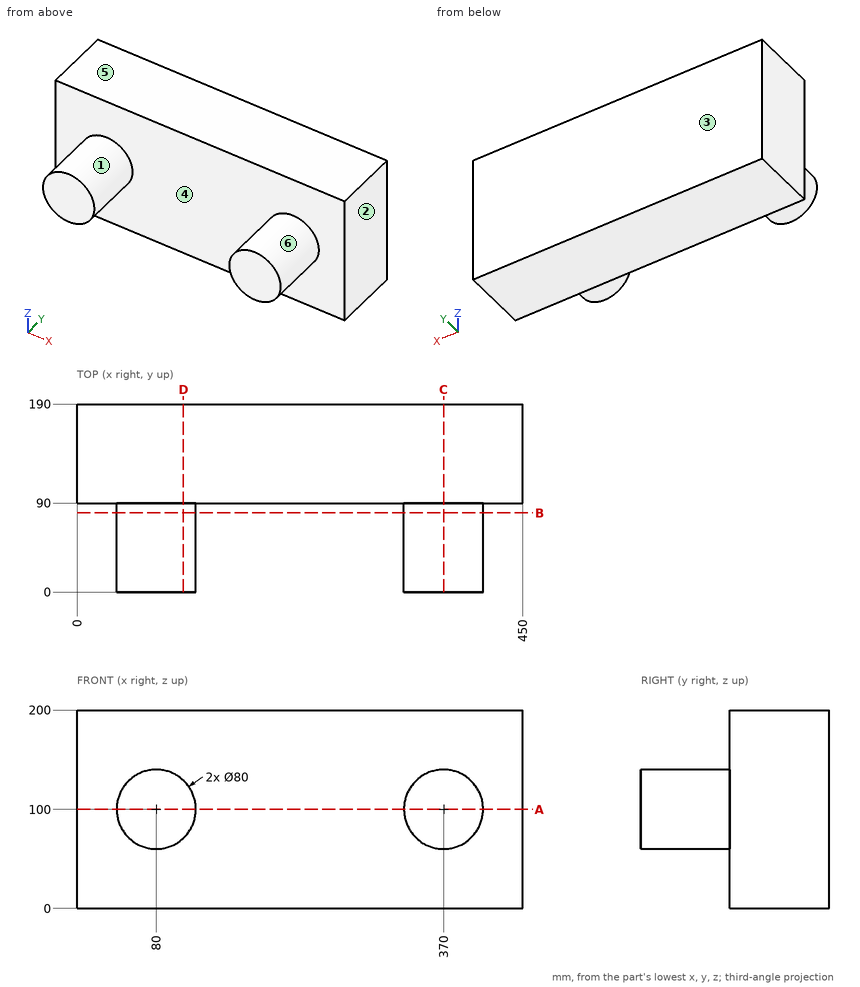
Answer from the drawing. Dimensions are ordinates in mm from the lowest x, y and z of the part. A direction names the side the tool comes from. Round coordinates to 2 decimals unless told otherwise and drop trailing zeros. Loops run counter-clockwise (first coordinate to the right, second up) from the corner with the lowest first, then second, coordinate; pieces in that order, holes last. Notation, with made-up numbers: (43, 38.25) - (60, 38.25) arc R32 ccw to (60, 76.25) - close; hole circle Ø9 at (-26, -37). An arc over 180 degrees is marked (long way). Return JSON: item names as keys, results as strings. Group by question number.
1. The part is cut by section B-B on y = 80. Determine the outline of the cut face in (x, z), then the cut area to 3 significant figures.
2. The mould has two halves that part along X. Classify the marked faces 1, 2, 3 and 4: pulls with the +X half, pulls with the -X half, needs draft (parallel to the pull), parting line crosses it, or undercut.
3. The part is cut by section D-D on x = 107.5. Determine the outline of the cut face in (y, z), then the cut area to 3 significant figures.
4. The part is cut by section C-C on x = 370. Determine the outline of the cut face in (y, z).
5. Consider probe 1 along Y at (x, z) = (151.5, 74.5); probe 2 along Z at (x, y) = (368.5, 44); probe 3 along X at (y, z) = (83, 83). Determine where each line is inside the solid, lowest interval first.
6. Which of the six approach directions +Z, -Z, +X, -X, +Y, -Y give full straight-line access (tool end or side, diameter ignored) to the marked faces 5 and 6?
7. The part is cut by section A-A on z = 100. Determine the outline of the cut face in (x, y), then the cut area to 3 significant figures.
Resolved:
{
 "1": {"outline": "circle Ø80 at (80, 100); circle Ø80 at (370, 100)", "area": "10,100 mm²"},
 "2": {"face 1": "undercut", "face 2": "pulls with the +X half", "face 3": "needs draft", "face 4": "undercut"},
 "3": {"outline": "(0, 70.95) - (90, 70.95) - (90, 0) - (190, 0) - (190, 200) - (90, 200) - (90, 129.05) - (0, 129.05) - close", "area": "25,200 mm²"},
 "4": {"outline": "(0, 60) - (90, 60) - (90, 0) - (190, 0) - (190, 200) - (90, 200) - (90, 140) - (0, 140) - close"},
 "5": {"probe 1": "y = 90 to 190", "probe 2": "z = 60.03 to 139.97", "probe 3": "x = 43.79 to 116.21, 333.79 to 406.21"},
 "6": {"face 5": "+Z, +X, -X, +Y, -Y", "face 6": "-Y"},
 "7": {"outline": "(0, 90) - (40, 90) - (40, 0) - (120, 0) - (120, 90) - (330, 90) - (330, 0) - (410, 0) - (410, 90) - (450, 90) - (450, 190) - (0, 190) - close", "area": "59,400 mm²"}
}
